```python
from build123d import *

# Parameters (mm, degrees)
SKETCH1_R            = 62.5
BOSS_EXTRUDE1_DEPTH  = 3.75
M6_CLEARANCE_HOLE1_D = 7
CIRPATTERN1_COUNT    = 2


with BuildPart() as part:
    # Sketch1 → Boss-Extrude1 (new body)
    with BuildSketch(Plane(origin=(0, 0, 0), x_dir=(1, 0, 0), z_dir=(0, 1, 0))):
        with Locations(Location((0, 0, 0), (0, 0, 270))):
            Circle(SKETCH1_R)
    extrude(amount=BOSS_EXTRUDE1_DEPTH)

    # M6 Clearance Hole1 (through all)
    with Locations(Plane(origin=(0, 3.75, 0), x_dir=(1, 0, 0), z_dir=(0, 1, 0))):
        with Locations((-54.4, 0)):
            m6_clearance_hole1 = Hole(M6_CLEARANCE_HOLE1_D / 2)

    # CirPattern1: M6 Clearance Hole1 ×2 about axis
    cirpattern1_axis = Axis((0, 0, 0), (0, 1, 0))
    for i in range(1, CIRPATTERN1_COUNT):
        add(m6_clearance_hole1.rotate(cirpattern1_axis, i * 360 / CIRPATTERN1_COUNT), mode=Mode.SUBTRACT)


solid = part.part
```
Model file for the job. Use its own axes, mm. Coordinates: 2 decimals unless noted, no trailing zeros. Loops run counter-clockwise (first coordinate to the right, second up) from the corner with the lowest first, then second, coordinate; pieces in that order, holes last. Notation, with made-up numbers: (81, -6.75) - (89, -6.75) arc R5 cw to (89, -1.75) - close; hole circle Ø1 at (-8, 50). An arc over 180 degrees is marked (long way). Answer as a JSON object with one key per item and string values. Group by question number.
(1) Cut at B-B (y = 0.85). Give the cut face in (x, z).
(2) Probe line 1 along Z through (x, y) = (54.4, 2.3); line 2 along Z through (x, y) = (57, 2.1); line 3 along Z through (x, y) = (1, 2.45). List the from-to ranges inside material, lowest first.
(3) Cut at C-C (x = 54.4). Give the cut face in (y, z).
(4) Cut at A-A (z = 0). Give the cut face in (x, y).
(5) Flat gauge pins, fed straight in: pin 1 (4 mm diameter, centred on x = -54.4, z = 0, fed in from -Y); pin 2 (12 mm diameter, centred on x = -10, z = -5.5, fed in from -Y). Where does each tip first touch, or does it go through?
(6) Two-plate mould, pull along X, no slides. Class faces 1 (the face through (1, 0, -1)), 2 (the face through (2.75, 1.85, -62.44)), 3 (the face through (51.6, 1.8, -2.1)): released by +X, released by -X, zero draft, split by the parting line, or undercut.
(7) Cut at D-D (x = 29). Give the cut face in (y, z).
Geometry says:
{
 "1": {"outline": "circle Ø125 at (0, 0); hole circle Ø7 at (-54.4, 0); hole circle Ø7 at (54.4, 0)"},
 "2": {"line 1": "z = -30.77 to -3.5, 3.5 to 30.77", "line 2": "z = -25.64 to -2.34, 2.34 to 25.64", "line 3": "z = -62.49 to 62.49"},
 "3": {"outline": "(0, -30.77) - (3.75, -30.77) - (3.75, -3.5) - (0, -3.5) - close; (0, 3.5) - (3.75, 3.5) - (3.75, 30.77) - (0, 30.77) - close"},
 "4": {"outline": "(-62.5, 0) - (-57.9, 0) - (-57.9, 3.75) - (-62.5, 3.75) - close; (-50.9, 0) - (50.9, 0) - (50.9, 3.75) - (-50.9, 3.75) - close; (57.9, 0) - (62.5, 0) - (62.5, 3.75) - (57.9, 3.75) - close"},
 "5": {"pin 1": "passes through", "pin 2": "stops at y = 0"},
 "6": {"face 1": "zero draft", "face 2": "split by the parting line", "face 3": "undercut"},
 "7": {"outline": "(0, -55.36) - (3.75, -55.36) - (3.75, 55.36) - (0, 55.36) - close"}
}
